Design review of the part shown in the three views and the two pictorial views. Dimensions are in mm from the part's minimum x, y and z. A direction names the side the tool comes from. Round coordinates to 2 decimals unless told otherwise and drop trailing zeros. Loops run counter-clockwise (first coordinate to the right, second up) from the corner with the lowest first, then second, coordinate; pieces in that order, holes last. Notation, with made-up numbers: M -19.75,-15 L -7.75,-15 A19 ccw -7.75,7 Z; hole C 56.5,-7.5 d10. An arc over 180 degrees is marked long. Answer in a Markdown table with one row per item. Add a question column.
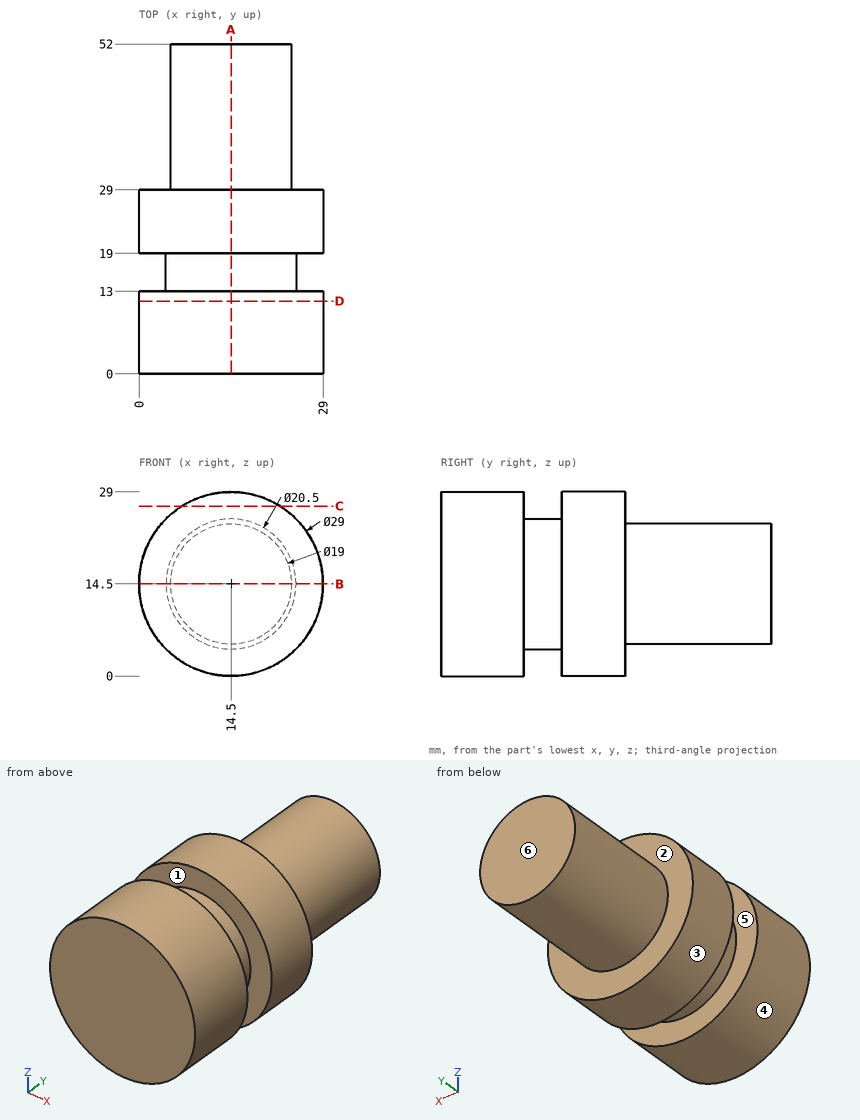
1. Take a section at A-A, the plane x = 14.5. State the section outline as (y, z) points, and give its area (3 significant figures).
2. Take a section at D-D, the plane y = 11.5. State the section outline as (x, z) points.
3. For pin 1 Ø3 at (x, y) = (24.5, 18) entering from +Z; pin 2 Ø4 at (x, y) = (22, 9.5) entering from +Z; pin 3 Ø4 at (y, z) = (21, 7.5) entering from +X, all flat-tipped, find the tip position at first contact; note any pin that passes through.
4. To check wall thickness, follow probe 1 along Y at (x, z) = (22.5, 8); probe 2 along X at (y, z) = (27.5, 4.25); probe 3 along Y at (x, z) = (8.5, 22.25). State the ranges of each line that lie inside material, in increasing order.
5. Machinability: for the marked faces 1, 2 and 3, which of the approach directions +Z, -Z, +X, -X, +Y, -Y give a long, thin tool a straight path to every point of the face, cutting with its end or side? Answer none if there is none.
6. Take a section at B-B, the plane z = 14.5. State the section outline as (x, y) points, and give its area (3 significant figures).
7. Take a section at C-C, the plane z = 26.75. State the section outline as (x, y) points.
8. Mouldability with a two-part tool opening along Y and no side actions: class the marked faces 4, 5 and 6 as released by +Y, released by -Y, zero draft, split by the parting line, or undercut.
Check sheet entries:
| question | item | result |
|---|---|---|
| 1 | outline | M 0,0 L 13,0 L 13,4.25 L 19,4.25 L 19,0 L 29,0 L 29,5 L 52,5 L 52,24 L 29,24 L 29,29 L 19,29 L 19,24.75 L 13,24.75 L 13,29 L 0,29 Z |
| 1 | area | 1,230 mm^2 |
| 2 | outline | C 14.5,14.5 d29 |
| 3 | pin 1 | stops at z = 25.96 |
| 3 | pin 2 | stops at z = 27.92 |
| 3 | pin 3 | stops at x = 28.11 |
| 4 | probe 1 | y = 0 to 13, 19 to 29 |
| 4 | probe 2 | x = 4.24 to 24.76 |
| 4 | probe 3 | y = 0 to 29 |
| 5 | face 1 | none |
| 5 | face 2 | +Y |
| 5 | face 3 | +Y, -Y |
| 6 | outline | M 0,0 L 29,0 L 29,13 L 24.75,13 L 24.75,19 L 29,19 L 29,29 L 24,29 L 24,52 L 5,52 L 5,29 L 0,29 L 0,19 L 4.25,19 L 4.25,13 L 0,13 Z |
| 6 | area | 1,230 mm^2 |
| 7 | outline | M 6.74,0 L 22.26,0 L 22.26,13 L 6.74,13 Z; M 6.74,19 L 22.26,19 L 22.26,29 L 6.74,29 Z |
| 8 | face 4 | zero draft |
| 8 | face 5 | undercut |
| 8 | face 6 | released by +Y |
